Drawing for the job (mm, zero at the part's lowest x, y, z). Round coordinates to 2 decimals unless told otherwise and drop trailing zeros. Write each loop counter-clockwise with the first axis right and the second up, starting at its lowest first coordinate (ties: lowest second). Pieces come first, ordered by that corner, then holes.
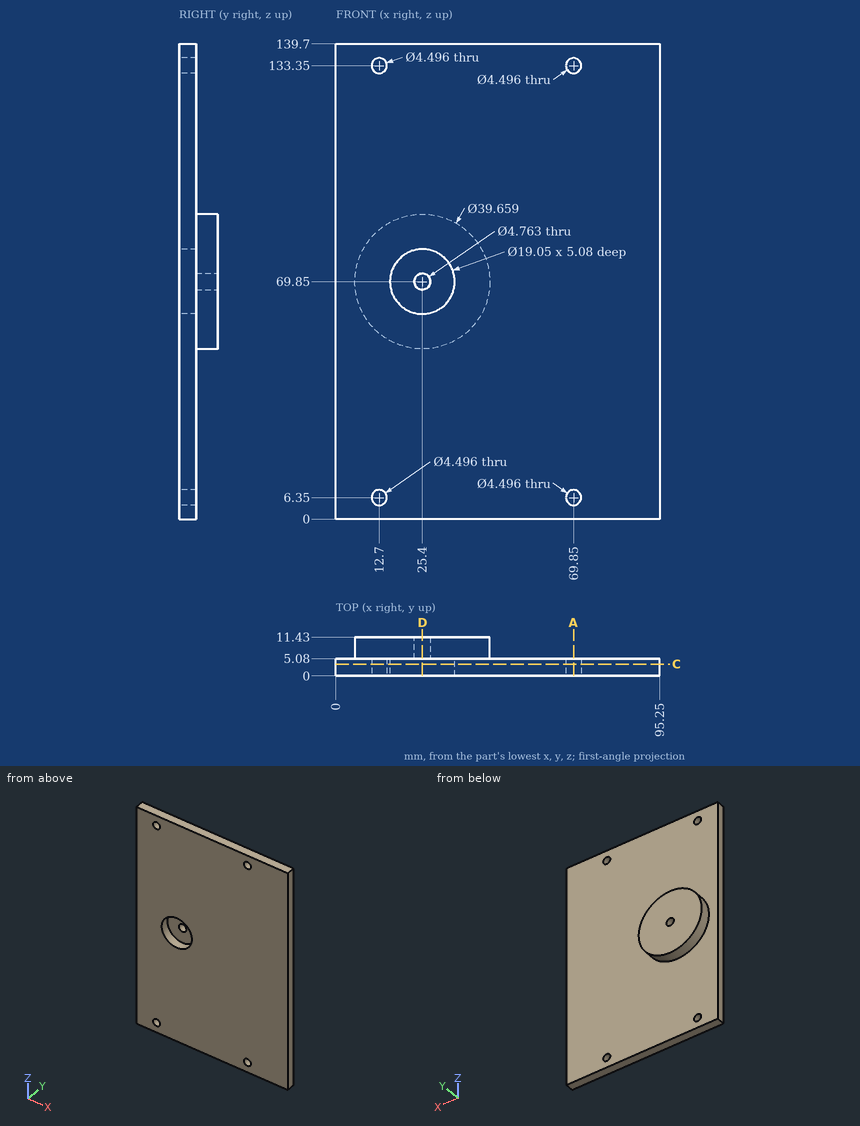
Q1. Saw through at D-D, the plane x = 25.4. Write the cut outline in (y, z) (1 decimal).
Q2. Wall check: line 1 (X direction, y = 4, z = 133.35); line 2 (Z direction, x = 25.4, y = 6.75); line 3 (Z direction, x = 69.85, y = 1.2). Give the ranges that are in metal, low to high.
Q3. Saw through at C-C, the plane y = 3.5. Give the number of separate pieces and of enclosed holes in the cut face, and give its area (3 significant figures).
Q4. Drop flat-ended pins along their axis: P1, Ø11.5, axis at x = 25.4, z = 69.85, coming from the -Y side; P2, Ø6, axis at x = 69.85, z = 133.35, coming from the +Y side. Give the stop position or say it passes through.
Q5. Saw through at A-A, the plane x = 69.85. Write the cut outline in (y, z), and give its area (3 significant figures).
Computed:
1. outline: (0, 0) - (5.1, 0) - (5.1, 50) - (11.4, 50) - (11.4, 67.5) - (5.1, 67.5) - (5.1, 60.3) - (0, 60.3) - close; (0, 79.4) - (5.1, 79.4) - (5.1, 72.2) - (11.4, 72.2) - (11.4, 89.7) - (5.1, 89.7) - (5.1, 139.7) - (0, 139.7) - close
2. line 1: x = 0 to 10.45, 14.95 to 67.6, 72.1 to 95.25
2. line 2: z = 50.02 to 67.47, 72.23 to 89.68
2. line 3: z = 0 to 4.1, 8.6 to 131.1, 135.6 to 139.7
3. separate pieces: 1
3. enclosed holes: 5
3. area: 13,000 mm2
4. P1: stops at y = 5.08
4. P2: stops at y = 5.08
5. outline: (0, 0) - (5.08, 0) - (5.08, 4.1) - (0, 4.1) - close; (0, 8.6) - (5.08, 8.6) - (5.08, 131.1) - (0, 131.1) - close; (0, 135.6) - (5.08, 135.6) - (5.08, 139.7) - (0, 139.7) - close
5. area: 664 mm2
